```python
from build123d import *

# Parameters (mm, degrees)
F2_DEPTH   = 12
F3_SIZE2   = 5
F3_SIZE    = 2
F3_2_SIZE2 = 5
F3_2_SIZE  = 2
F4_R       = 3


with BuildPart() as f2:
    # F1 (on Top) → F2 (new body)
    with BuildSketch(Plane.XY):
        with BuildLine():
            Line((15, 3.5), (15, 15))
            Line((15, 15), (-15, 15))
            Line((-15, 15), (-15, -15))
            Line((-15, -15), (15, -15))
            Line((15, -15), (15, -3.5))
            Line((15, -3.5), (-2, -3.5))
            ThreePointArc((-2, -3.5), (-5.5, 0), (-2, 3.5))
            Line((-2, 3.5), (15, 3.5))
        make_face()
    extrude(amount=F2_DEPTH)

    # F3
    f3_edges = [f2.edges().sort_by_distance(p)[0] for p in [
        (15, -9.25, 12),
    ]]
    f3_side = f2.faces().sort_by_distance((15, -9.25, 6))[0]
    chamfer(f3_edges, length=F3_SIZE, length2=F3_SIZE2, reference=f3_side)

    # F3#2
    f3_2_edges = [f2.edges().sort_by_distance(p)[0] for p in [
        (15, 9.25, 12),
    ]]
    f3_2_side = f2.faces().sort_by_distance((15, 9.25, 6))[0]
    chamfer(f3_2_edges, length=F3_2_SIZE, length2=F3_2_SIZE2, reference=f3_2_side)

    # F4
    f4_edges = [f2.edges().sort_by_distance(p)[0] for p in [
        (-15, -15, 6),
        (15, -15, 5),
        (15, 15, 5),
        (-15, 15, 6),
        (15, -3.5, 5),
        (15, 3.5, 5),
    ]]
    fillet(f4_edges, radius=F4_R)


solid = f2.part
```
CAD build for the part. Positions are in the model's coordinates, mm. A direction names the side the tool comes from. Coordinates: 2 decimals unless noted, no trailing zeros. Write each loop counter-clockwise with the first axis right and the second up, starting at its lowest first coordinate (ties: lowest second). Pieces come first, ordered by that corner, then holes.
(1) Cut at B-B, the plane z = 8.25. List the corners of the cut face in (x, y), and give its area (3 significant figures).
(2) Cut at C-C, the plane y = 6. List the corners of the cut face in (x, z).
(3) Drill centre lines: probe 1 along Y at (x, z) = (9, 5.25); probe 2 along X at (y, z) = (-0.25, 5.25); probe 3 along Z at (x, y) = (12, -6.25). Where is each one in solid material? Low to high.
(4) Cut at A-A, the plane x = -0.5. List the corners of the cut face in (y, z).
(5) Cut at D-D, the plane z = 10.75. List the corners of the cut face in (x, y) (3 decimals), and give its area (3 significant figures).
(6) Flat gauge pin, fed straight in: pin 1 (3 mm diameter, centred on x = 4, y = 1.5, fed in from -Z). Where does the tip first touch, or does it go through?
(7) 3-axis set-ups, long thin cutter, end or side, ignore diameter. For faces 4 (the face through (0, 4, 0)), 5 (the face through (5, -3.5, 6)): which of +Z, -Z, +X, -X, +Y, -Y reach the whole face in a straight line?
(8) Two-plate mould, pull along Y, no slides. Class faces 1 (the face through (14.1, -14.14, 5.68)), 2 (the face through (5, 3.5, 6)), 3 (the face through (12.5, 9.2, 11)): +Y half, -Y half, draft (parallel to the pull), parting line (faces both ways), or undercut.
Geometry says:
1. outline: (-15, -12) arc R3 ccw to (-12, -15) - (12, -15) arc R3 ccw to (15, -12) - (15, -6.5) arc R3 ccw to (12, -3.5) - (-2, -3.5) arc R3.5 cw to (-2, 3.5) - (12, 3.5) arc R3 ccw to (15, 6.5) - (15, 12) arc R3 ccw to (12, 15) - (-12, 15) arc R3 ccw to (-15, 12) - close
1. area: 750 mm2
2. outline: (-15, 0) - (14.96, 0) - (14.96, 10.02) - (10, 12) - (-15, 12) - close
3. probe 1: y = -15 to -3.5, 3.5 to 15
3. probe 2: x = -15 to -5.49
3. probe 3: z = 0 to 11.2
4. outline: (-15, 0) - (-3.5, 0) - (-3.5, 12) - (-15, 12) - close; (3.5, 0) - (15, 0) - (15, 12) - (3.5, 12) - close
5. outline: (-15, -12) arc R3 ccw to (-12, -15) - (12, -15) arc R3 ccw to (13.125, -14.781) - (13.125, -3.719) arc R3 ccw to (12, -3.5) - (-2, -3.5) arc R3.5 cw to (-2, 3.5) - (12, 3.5) arc R3 ccw to (13.125, 3.719) - (13.125, 14.781) arc R3 ccw to (12, 15) - (-12, 15) arc R3 ccw to (-15, 12) - close
5. area: 714 mm2
6. pin 1: passes through
7. face 4: -Z, +X, -X, +Y, -Y
7. face 5: +Z, -Z, +X
8. face 1: -Y half
8. face 2: undercut
8. face 3: draft
